Check sheet for the modelled part. Datum: model origin and axes. Units: mm. Face numbers are marked on the shaded views. A direction names the side the tool comes from. Coordinates: 2 decimals unless noted, no trailing zeros. Write each loop counter-clockwise with the first axis right and the second up, starting at its lowest first coordinate (ties: lowest second). Pieces come first, ordered by that corner, then holes. Notation, with made-up numbers: M 81.25,50.5 L 91.25,50.5 A23 cw 91.25,77.5 Z; hole C -34.5,8 d3. An arc over 180 degrees is marked long. Answer as CSV lines item,"result". Start each with the question number.
Q1. Sectioned sample at A-A, the plane x = 0. Record the cut outline in (y, z).
Q2. Depth check by flat-ended pin: pin 1 Ø4 at (y, z) = (-2.5, 5) entering from +X; pin 2 Ø8 at (y, z) = (-2.5, 14) entering from -X; pin 3 Ø6 at (x, z) = (-0.5, 5) entering from -Y. Enter the tip coordinate at first touch or a pass-through.
Q3. Sectioned sample at D-D, the plane z = 14.5. Record the cut outline in (x, y), then the cut area to 3 significant figures.
Q4. Sectioned sample at C-C, the plane z = 3.25. Record the cut outline in (x, y).
Q5. Thickness scan on line 1 along Z through (x, y) = (6.75, 2.25); line 2 along X through (y, z) = (0, 14.5); line 3 along Y through (x, z) = (1.75, 5). Record the ranges inside material, lowest first. Write a range as from..to.
Q6. Access from +Z, -Z, +X, -X, +Y, -Y to the whole of each face (thin tool, end or side, straight path). Record for the marked faces 1 and 2.
Solid Edge part; units mm, degrees
sketch "Sketch1" plane through (0, 0, 0) normal (1, 0, 0) x (0, 1, 0)
  line L0 (9.5, 25) -> (9.5, 24)
  line L1 (9.5, 24) -> (8, 24)
  line L2 (8, 24) -> (8, 10)
  line L3 (8, 10) -> (6.75, 10)
  line L4 (6.75, 10) -> (6.75, 0)
  line L5 (6.75, 0) -> (0, 0)
  line L6 (0, 26) -> (9, 26)
  line L7 (9, 26) -> (9.5, 25)
  dimension "D1" = 9.5
  dimension "D2" = 9
revolve "RevolvedProtrusion1" add sketch "Sketch1" angle 360 about axis through (0, 0, 0) along (0, 0, 1)
properties material "Stainless steel"
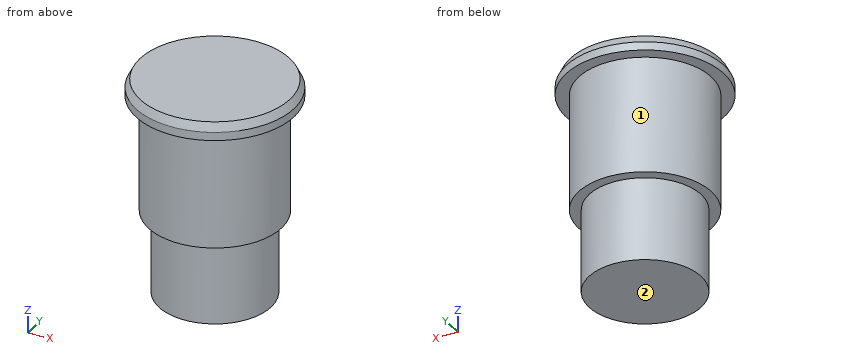
Output:
1,outline,"M -9.5,24 L -8,24 L -8,10 L -6.75,10 L -6.75,0 L 6.75,0 L 6.75,10 L 8,10 L 8,24 L 9.5,24 L 9.5,25 L 9,26 L -9,26 L -9.5,25 Z"
2,pin 1,"stops at x = 6.73"
2,pin 2,"stops at x = -8"
2,pin 3,"stops at y = -6.75"
3,outline,"C 0,0 d16"
3,area,"201 mm^2"
4,outline,"C 0,0 d13.5"
5,line 1,"z = 10..26"
5,line 2,"x = -8..8"
5,line 3,"y = -6.52..6.52"
6,face 1,"-Z"
6,face 2,"-Z, +X, -X, +Y, -Y"
